Study the drawing (mm; zero at the part's minimum x, y, z) and answer. A direction names the side the tool comes from. Coordinates: 2 decimals unless noted, no trailing zeros. Order: outer loops, then holes, each group sorted by start corner. A loop starts at its lowest first (then second) coordinate and runs counter-clockwise, first axis right, second up.
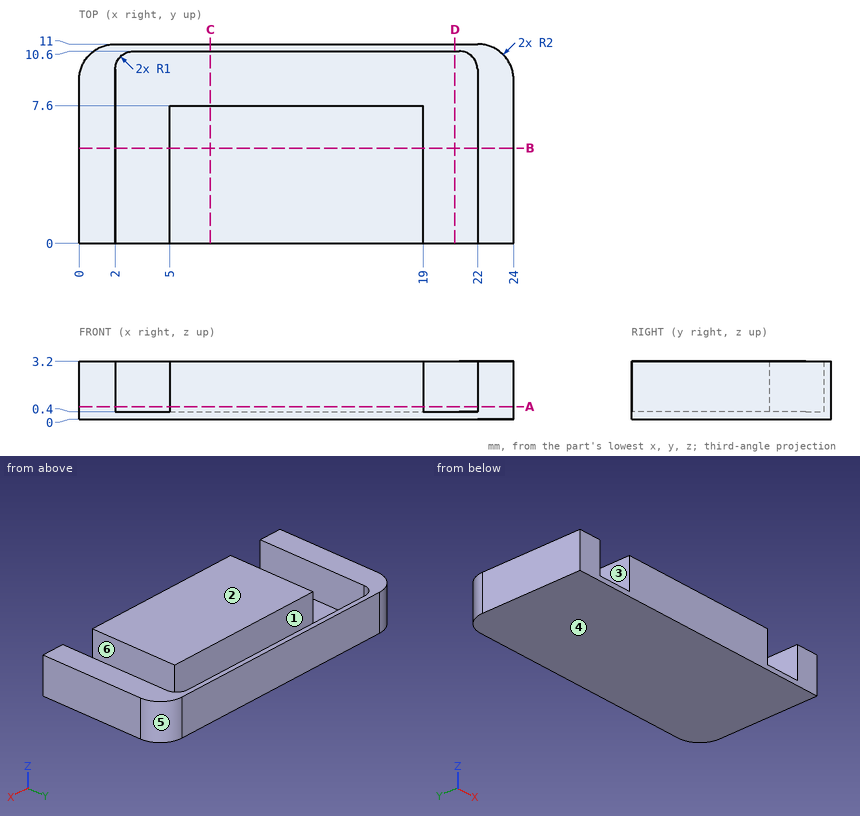
1) A cutting plane is placed at B-B, the plane y = 5.25. Determine the outline of the cut face in (x, z), and give its area (3 significant figures).
A:
outline: (0, 0) - (24, 0) - (24, 3.2) - (22, 3.2) - (22, 0.4) - (19, 0.4) - (19, 3.2) - (5, 3.2) - (5, 0.4) - (2, 0.4) - (2, 3.2) - (0, 3.2) - close
area: 60.0 mm2
2) Straight lines are drawn through the part: line 1 (X direction, y = 0.5, z = 1.3); line 2 (Y direction, x = 15.5, z = 1.4); line 3 (X direction, y = 8.75, z = 0.85). For each, find the intervals that lie inside material, in ascending order.
A:
line 1: x = 0 to 2, 5 to 19, 22 to 24
line 2: y = 0 to 7.6, 10.6 to 11
line 3: x = 0 to 2, 22 to 24
3) A cutting plane is placed at D-D, the plane x = 20.75. Determine the outline of the cut face in (y, z), and give its area (3 significant figures).
A:
outline: (0, 0) - (11, 0) - (11, 3.2) - (10.6, 3.2) - (10.6, 0.4) - (0, 0.4) - close
area: 5.52 mm2
4) Determine the mould class of the marked faces 4, 5 and 6 for opening direction X: pulls with the +X half, pulls with the -X half, needs draft (parallel to the pull), parting line crosses it, or undercut.
A:
face 4: needs draft
face 5: pulls with the +X half
face 6: undercut
5) A cutting plane is placed at A-A, the plane z = 0.7. Determine the outline of the cut face in (x, y), and give its area (3 significant figures).
A:
outline: (0, 0) - (2, 0) - (2, 9.6) arc R1 cw to (3, 10.6) - (21, 10.6) arc R1 cw to (22, 9.6) - (22, 0) - (24, 0) - (24, 9) arc R2 ccw to (22, 11) - (2, 11) arc R2 ccw to (0, 9) - close; (5, 0) - (19, 0) - (19, 7.6) - (5, 7.6) - close
area: 157 mm2
6) A cutting plane is placed at C-C, the plane x = 7.25. Determine the outline of the cut face in (y, z).
A:
outline: (0, 0) - (11, 0) - (11, 3.2) - (10.6, 3.2) - (10.6, 0.4) - (7.6, 0.4) - (7.6, 3.2) - (0, 3.2) - close
7) Which of the six approach directions +Z, -Z, +X, -X, +Y, -Y give full straight-line access (tool end or side, diameter ignored) to the marked faces 1, 2 and 3?
A:
face 1: +Z
face 2: +Z, +X, -X, +Y, -Y
face 3: +Z, -Y
